Job drawing, mm, ordinate dimensions from the low corner. One solid piece. A direction names the side the tool comes from. Coordinates: 2 decimals unless noted, no trailing zeros. Order: outer loops, then holes, each group sorted by start corner. A loop starts at its lowest first (then second) coordinate and runs counter-clockwise, first axis right, second up. Notation, with made-up numbers: M -15,12 L 28,12 A10 cw 28,19 Z; hole C -6,-1.75 d1. An arc over 180 degrees is marked long. Write item = value, one per line.
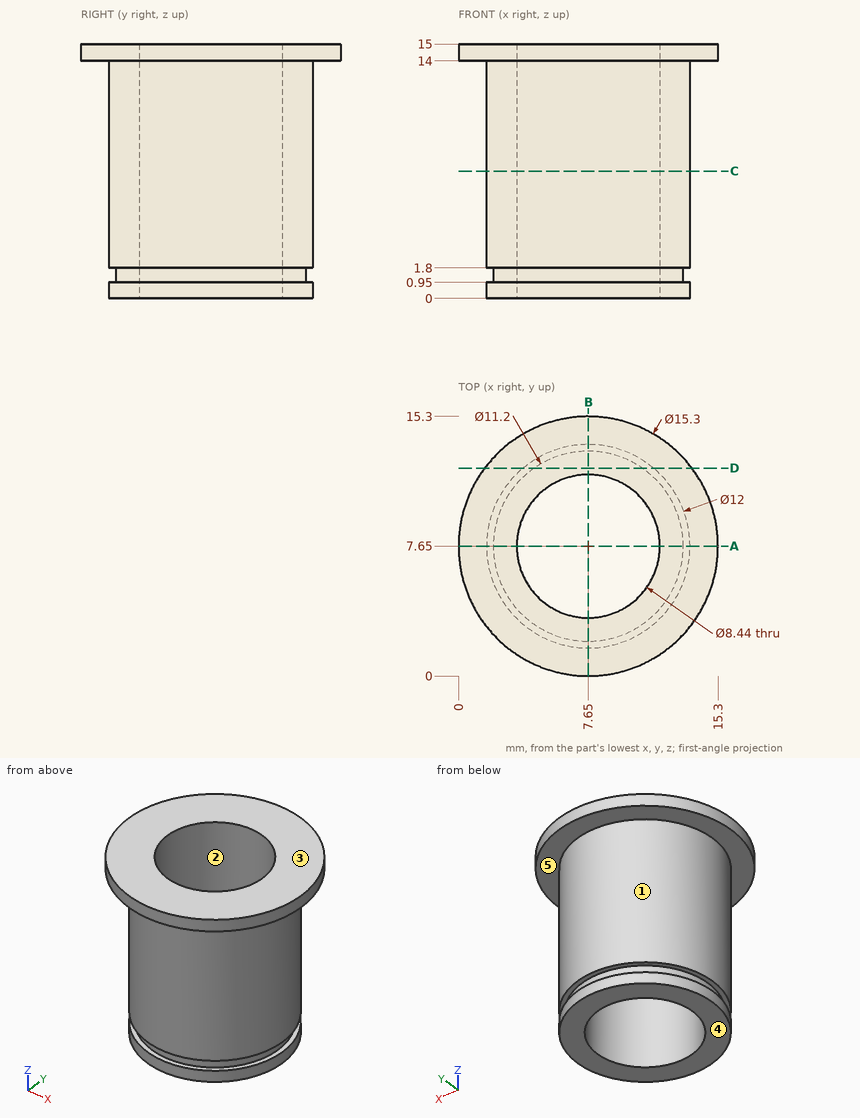
(1) Slice it at D-D, the plane y = 12.25. Write the cut outline in (x, z).
Evaluation:
outline = M 1.54,14 L 3.8,14 L 3.8,1.8 L 4.46,1.8 L 4.46,0.95 L 3.8,0.95 L 3.8,0 L 11.5,0 L 11.5,0.95 L 10.84,0.95 L 10.84,1.8 L 11.5,1.8 L 11.5,14 L 13.76,14 L 13.76,15 L 1.54,15 Z
(2) Pull direction X, two halves, no side cores. Call the marked faces 1, 2 and 3: +X half, -X half, draft (parallel to the pull), parting line (faces both ways), or undercut.
Evaluation:
face_1 = parting line
face_2 = undercut
face_3 = draft
(3) Pin check, flat tips, straight feed: pin 1 Ø8 at (x, z) = (7, 7) entering from +Y; pin 2 Ø7 at (x, y) = (7.65, 7.65) entering from -Z; pin 3 Ø2 at (x, z) = (6.5, 3) entering from -Y. Stop position of each tip, or through.
Evaluation:
pin_1 = 13.65
pin_2 = through
pin_3 = 1.65
(4) Wall check: line 1 (Z direction, x = 13, y = 5.5); line 2 (Z direction, x = 12.75, y = 11.5); line 3 (Y direction, x = 8.5, z = 8). Give the ranges that are in metal, low to high. Write a range as from..to.
Evaluation:
line_1 = 0..0.95, 1.8..15
line_2 = 14..15
line_3 = 1.71..3.52, 11.78..13.59
(5) Slice it at C-C, the plane z = 7.5. Write the cut outline in (x, y).
Evaluation:
outline = C 7.65,7.65 d12; hole C 7.65,7.65 d8.44
(6) Slice it at A-A, the plane y = 7.65. Write the cut outline in (x, z), then the cut area to 3 significant figures.
Evaluation:
outline = M 0,14 L 1.65,14 L 1.65,1.8 L 2.05,1.8 L 2.05,0.95 L 1.65,0.95 L 1.65,0 L 3.43,0 L 3.43,15 L 0,15 Z; M 11.87,0 L 13.65,0 L 13.65,0.95 L 13.25,0.95 L 13.25,1.8 L 13.65,1.8 L 13.65,14 L 15.3,14 L 15.3,15 L 11.87,15 Z
area = 56.0 mm²
(7) Tool access for the marked faces 4 and 5: list every direction of +Z, -Z, +X, -X, +Y, -Y with a clear straight run to the whole face (end or side of a thin tool).
Evaluation:
face_4 = -Z, +X, -X, +Y, -Y
face_5 = -Z
